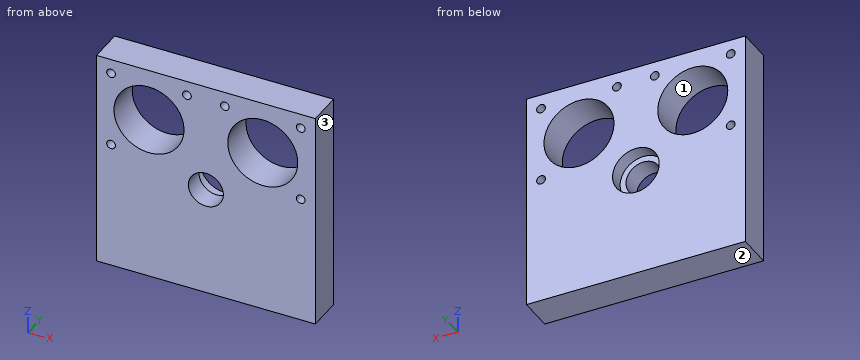
```python
from build123d import *

# Parameters (mm, degrees)
F0_W     = 75
F0_H     = 75
F1_DEPTH = 6
F2_R     = 12
F2_R_2   = 1.5
F3_DEPTH = 12.001
F4_R     = 8
F5_DEPTH = 5
F6_R     = 6
F7_DEPTH = 7.001


with BuildPart() as f1:
    # F0 (on Front) → F1 (new body, symmetric)
    with BuildSketch(Plane.XZ):
        Rectangle(F0_W, F0_H)
    extrude(amount=F1_DEPTH, both=True)

    # F2 (on face) → F3 (cut, through all)
    with BuildSketch(Plane(origin=(0, 6, 0), x_dir=(-1, 0, 0), z_dir=(0, 1, 0))):
        with Locations((-19.5, 19.5)):
            Circle(F2_R)
        with Locations((-32.5, 32.5)):
            Circle(F2_R_2)
        with Locations((-32.5, 6.5)):
            Circle(F2_R_2)
        with Locations((-6.5, 32.5)):
            Circle(F2_R_2)
        with Locations((32.5, 6.5)):
            Circle(F2_R_2)
        with Locations((32.5, 32.5)):
            Circle(F2_R_2)
        with Locations((19.5, 19.5)):
            Circle(F2_R)
        with Locations((6.5, 32.5)):
            Circle(F2_R_2)
    extrude(amount=-F3_DEPTH, mode=Mode.SUBTRACT)

    # F4 (on face) → F5 (cut)
    with BuildSketch(Plane(origin=(0, 6, 0), x_dir=(-1, 0, 0), z_dir=(0, 1, 0))):
        Circle(F4_R)
    extrude(amount=-F5_DEPTH, mode=Mode.SUBTRACT)

    # F6 (on face) → F7 (cut, through all)
    with BuildSketch(Plane(origin=(0, 1, 0), x_dir=(-1, 0, 0), z_dir=(0, 1, 0))):
        Circle(F6_R)
    extrude(amount=-F7_DEPTH, mode=Mode.SUBTRACT)


solid = f1.part
```
Build history of the part. All positions in model axes, mm. Face numbers are marked on the shaded views. Round coordinates to 2 decimals unless told otherwise and drop trailing zeros. Loops run counter-clockwise (first coordinate to the right, second up) from the corner with the lowest first, then second, coordinate; pieces in that order, holes last.
Item 1: Two-plate mould, pull along Z, no slides. Class the marked faces 1, 2 and 3: released by +Z, released by -Z, zero draft, split by the parting line, or undercut.
Item 2: Saw through at A-A (z = 0). List the corners of the cut face in (x, y).
Item 3: Saw through at B-B (y = -1.5). State how many separate pieces and enclosed holes the cut face has, then the cut area to 3 significant figures.
Item 4: Pin check, flat tip, straight feed: P1, Ø15.5, axis at x = 0, z = 0, coming from the +Y side. Stop position of the tip, or through.
Item 5: Saw through at D-D (x = 0). List the corners of the cut face in (y, z), then the cut area to 3 significant figures.
Item 6: Drill centre lines: line 1 along Z through (x, y) = (32.5, 2); line 2 along X through (y, z) = (5.25, 10); line 3 along X through (y, z) = (2, 26). Where is each one in solid material? Low to high.
Item 7: Saw through at C-C (z = 19.5). List the corners of the cut face in (x, y), then the cut area to 3 significant figures.
Worked answers:
1. face 1: undercut
1. face 2: released by -Z
1. face 3: zero draft
2. outline: (-37.5, -6) - (-6, -6) - (-6, 1) - (-8, 1) - (-8, 6) - (-37.5, 6) - close; (6, -6) - (37.5, -6) - (37.5, 6) - (8, 6) - (8, 1) - (6, 1) - close
3. separate pieces: 1
3. enclosed holes: 9
3. area: 4,560 mm2
4. P1: stops at y = 1
5. outline: (-6, -37.5) - (6, -37.5) - (6, -8) - (1, -8) - (1, -6) - (-6, -6) - close; (-6, 6) - (1, 6) - (1, 8) - (6, 8) - (6, 37.5) - (-6, 37.5) - close
5. area: 736 mm2
6. line 1: z = -37.5 to 5, 8 to 31, 34 to 37.5
6. line 2: x = -37.5 to -26.83, -12.17 to 12.17, 26.83 to 37.5
6. line 3: x = -37.5 to -29.59, -9.41 to 9.41, 29.59 to 37.5
7. outline: (-37.5, -6) - (-31.5, -6) - (-31.5, 6) - (-37.5, 6) - close; (-7.5, -6) - (7.5, -6) - (7.5, 6) - (-7.5, 6) - close; (31.5, -6) - (37.5, -6) - (37.5, 6) - (31.5, 6) - close
7. area: 324 mm2
